Model file for the job. Use its own axes, mm. Round coordinates to 2 decimals unless told otherwise and drop trailing zeros. Answer as a JSON object with one key per item and string values.
Autodesk Inventor part; units mm, degrees
ref_plane "YZ Plane" through (0, 0, 0) normal (1, 0, 0) x (0, 1, 0)
ref_plane "XZ Plane" through (0, 0, 0) normal (0, 1, 0) x (-1, 0, 0)
ref_plane "XY Plane" through (0, 0, 0) normal (0, 0, 1) x (1, 0, 0)
sketch "Sketch1" plane through (0, 0, 0) normal (0, 1, 0) x (-1, 0, 0)
  line L0 (28.3692, 74.6141) -> (-56.6308, 74.6141)
  line L1 (-56.6308, 74.6141) -> (-56.6308, -415.3859)
  line L2 (-56.6308, -415.3859) -> (28.3692, -415.3859)
  line L3 (28.3692, -415.3859) -> (28.3692, 74.6141)
  point P0 (0, 0)
  dimension "d0" = 85
  dimension "d1" = 490
extrude "Extrusion1" add sketch "Sketch1" along normal blind 15
sketch "Sketch2" plane through (-28.3692, 0, 74.6141) normal (0, 0, 1) x (1, 0, 0)
  line L0 (85, 0) -> (0, 0)
  line L1 (0, 0) -> (85, 0)
  line L2 (85, 0) -> (85, 5)
  line L3 (85, 5) -> (0, 5)
  line L4 (0, 5) -> (0, 0)
  point P0 (28.3692, 0)
  dimension "d4" = 85
  dimension "d5" = 5
extrude "Extrusion2" cut sketch "Sketch2" against normal blind 7
sketch "Sketch3" plane through (56.6308, 0, -415.3859) normal (0, 0, -1) x (-1, 0, 0)
  line L0 (85, 0) -> (85, 15)
  line L1 (85, 5) -> (0, 5)
  line L2 (85, 0) -> (0, 0)
  line L3 (0, 0) -> (0, 5)
  line L4 (0, 5) -> (85, 5)
  line L5 (85, 5) -> (85, 0)
  point P0 (56.6308, 0)
  dimension "d8" = 85
  dimension "d9" = 5
extrude "Extrusion3" cut sketch "Sketch3" against normal blind 7
sketch "Sketch4" plane through (0, 0, 0) normal (0, -1, 0) x (1, 0, 0)
  line L0 (-28.3692, -408.3859) -> (56.6308, -408.3859)
  line L1 (56.6308, 67.6141) -> (56.6308, -408.3859)
  line L2 (56.6308, 67.6141) -> (-28.3692, 67.6141)
  line L3 (-28.3692, -408.3859) -> (-28.3692, 67.6141)
  line L4 (-28.3692, 67.6141) -> (56.6308, 67.6141)
  line L5 (-28.3692, -408.3859) -> (-28.3692, 67.6141)
  line L6 (56.6308, 67.6141) -> (-28.3692, 67.6141)
  line L7 (-28.3692, 67.6141) -> (-28.3692, -408.3859)
  line L8 (-28.3692, -408.3859) -> (56.6308, -408.3859)
  line L9 (56.6308, -408.3859) -> (56.6308, 67.6141)
  point P0 (0, 0)
extrude "Extrusion4" add sketch "Sketch4" along normal blind 1
properties part number "Arcade_top"
1) Probe probe 1 along Z at (x, y) = (-16, 4.25). List the from-to ranges inside material, lowest first.
Values follow:
{"probe 1": "-408.39 to 67.61"}
2) Drop a flat-ended pin along its axis: P1, Ø3.5, axis at x = 23.5, z = -413.5, coming from the -Y side. Give the stop position or say it passes through.
Values follow:
{"P1": "y = 5"}
3) Two-plate mould, pull along X, no slides. Class faces 1 (the flat face through (56.631, 7, -167)), 2 (the flat face through (15, 15, -167)), 3 (the flat face through (-28.369, 7, -174)): pulls with the +X half, pulls with the -X half, needs draft (parallel to the pull), parting line crosses it, or undercut.
Values follow:
{"face 1": "pulls with the +X half", "face 2": "needs draft", "face 3": "pulls with the -X half"}
